from build123d import *

# Parameters (mm, degrees)
F1_DEPTH  = 25.4
F2_W      = 31.608661
F2_H      = 81.88197
F3_DEPTH  = 50.8
F5_DEPTH  = 76.2
F6_W      = 15.80433
F6_H      = 18.276912
F8_W      = 15.80433
F8_H      = 18.276912
F10_R     = 8.263527
F11_DEPTH = 135.636


with BuildPart() as f1:
    # F0 (on Top) → F1 (new body)
    with BuildSketch(Plane.XY):
        with BuildLine():
            Line((45.138903, 75.711831), (26.379006, 75.711831))
            ThreePointArc((26.379006, 75.711831), (-0.25221, 49.080616), (-26.883425, 75.711831))
            Line((-26.883425, 75.711831), (-45.643322, 75.711831))
            Line((-45.643322, 75.711831), (-45.643322, -76.136142))
            Line((-45.643322, -76.136142), (-26.182505, -76.136142))
            ThreePointArc((-26.182505, -76.136142), (-0.25221, -50.205846), (25.678086, -76.136142))
            Line((25.678086, -76.136142), (45.138903, -76.136142))
            Line((45.138903, -76.136142), (45.138903, 75.711831))
        make_face()
        with BuildLine():
            ThreePointArc((-26.883425, 75.711831), (-0.25221, 102.343047), (26.379006, 75.711831))
            Line((26.379006, 75.711831), (45.138903, 75.711831))
            ThreePointArc((45.138903, 75.711831), (-0.25221, 121.102944), (-45.643322, 75.711831))
            Line((-45.643322, 75.711831), (-26.883425, 75.711831))
        make_face()
        with BuildLine():
            ThreePointArc((-45.643322, -76.136142), (-0.25221, -121.527255), (45.138903, -76.136142))
            Line((45.138903, -76.136142), (25.678086, -76.136142))
            ThreePointArc((25.678086, -76.136142), (-0.25221, -102.066438), (-26.182505, -76.136142))
            Line((-26.182505, -76.136142), (-45.643322, -76.136142))
        make_face()
    extrude(amount=F1_DEPTH)

    # F2 (on Top) → F3 (join)
    with BuildSketch(Plane.XY):
        with Locations((0.401416, -2.476901)):
            Rectangle(F2_W, F2_H)
    extrude(amount=F3_DEPTH)

    # F4 (on face) → F5 (cut)
    with BuildSketch(Plane.YZ.offset(16.205747)):
        with BuildLine():
            ThreePointArc((-25.140974, 50.8), (-2.476901, 28.135927), (20.187172, 50.8))
            Line((20.187172, 50.8), (-25.140974, 50.8))
        make_face()
        with BuildLine():
            Line((-25.140974, 50.8), (20.187172, 50.8))
            ThreePointArc((20.187172, 50.8), (-2.476901, 73.464073), (-25.140974, 50.8))
        make_face()
    extrude(amount=-F5_DEPTH, mode=Mode.SUBTRACT)

    # F6 (on face) → F7 (revolve)
    with BuildSketch(Plane.XY.offset(50.8)):
        with Locations((-7.500749, -34.27943)):
            Rectangle(F6_W, F6_H)
    revolve(axis=Axis((0.401416, -34.27943, 50.8), (0, -1, 0)))

    # F8 (on face) → F9 (revolve)
    with BuildSketch(Plane.XY.offset(50.8)):
        with Locations((-7.500749, 29.325628)):
            Rectangle(F8_W, F8_H)
    revolve(axis=Axis((0.401416, 29.325628, 50.8), (0, -1, 0)))

    # F10 (on face) → F11 (cut)
    with BuildSketch(Plane(origin=(0, 38.464084, 0), x_dir=(-1, 0, 0), z_dir=(0, 1, 0))):
        with Locations((-0.401416, 50.8)):
            Circle(F10_R)
    extrude(amount=-F11_DEPTH, mode=Mode.SUBTRACT)


solid = f1.part
The listing builds one solid part. Answer for the finished solid, in the listing's coordinates (mm). A direction names the side the tool comes from. Give positions to 0.01 mm unless a question says otherwise; leave off trailing zeros. Write each loop counter-clockwise with the first axis right and the second up, starting at its lowest first coordinate (ties: lowest second). Pieces come first, ordered by that corner, then holes.
Item 1: Section B-B, the plane x = 23 is taken. Write down the section's boundary in (y, z) (3 decimals), plus the area to 3 significant figures.
Item 2: Section D-D, the plane z = 55.5 is taken. Write down the section's boundary in (x, y).
Item 3: Determine the mould class of faces 1 (the flat face through (-1, 1, 0)), 2 (the cylindrical face through (0.75, 121.09, 12.52)), 3 (the cylindrical face through (5.521, 49.714, 12.522)) for opening direction Y: released by +Y, released by -Y, zero draft, split by the parting line, or undercut.
Item 4: Flat-ended cylindrical pins translate along their axes: P1, Ø12.5, axis at x = -1, z = 55.5, coming from the -Y side; P2, Ø12.5, axis at x = -5.5, z = 57.5, coming from the +Y side; P3, Ø4, axis at x = 7.5, y = -35, coming from the +Z side. Find the tip coordinate at first contact, or state that the pin passes through.
Item 5: Section C-C, the plane y = -86 is taken. Write down the section's boundary in (x, z), plus the area to 3 significant figures.
Item 6: Find the intervals of material crossed by line 1 along Y through (x, z) = (0.5, 60.5); line 2 along X through (y, z) = (27, 50.8); line 3 along Z through (x, y) = (1, 24.5), in increasing order.
Item 7: Which of the six approach directions +Z, -Z, +X, -X, +Y, -Y give full straight-line access (tool end or side, diameter ignored) to faces 4 (the flat face through (-15.403, -3, 27)), 5 (the flat face through (1, 20.187, 60)), 6 (the flat face through (16.206, -3, 27))?
Item 8: Section A-A, the plane z = 33.5 is taken. Write down the section's boundary in (x, y), plus the area to 3 significant figures.
Completed:
1. outline: (-115.119, 0) - (-87.613, 0) - (-87.613, 25.4) - (-115.119, 25.4) - close; (-64.659, 0) - (62.729, 0) - (62.729, 25.4) - (-64.659, 25.4) - close; (88.695, 0) - (114.695, 0) - (114.695, 25.4) - (88.695, 25.4) - close
1. area: 4,590 mm2
2. outline: (-14.69, -43.42) - (-6.4, -43.42) - (-6.4, -25.14) - (-14.69, -25.14) - close; (-14.69, 20.19) - (-6.4, 20.19) - (-6.4, 38.46) - (-14.69, 38.46) - close; (7.2, -43.42) - (15.49, -43.42) - (15.49, -25.14) - (7.2, -25.14) - close; (7.2, 20.19) - (15.49, 20.19) - (15.49, 38.46) - (7.2, 38.46) - close
3. face 1: zero draft
3. face 2: released by +Y
3. face 3: undercut
4. P1: stops at y = -43.42
4. P2: stops at y = 38.46
4. P3: stops at z = 65.76
5. outline: (-44.56, 0) - (-24.23, 0) - (-24.23, 25.4) - (-44.56, 25.4) - close; (23.73, 0) - (44.05, 0) - (44.05, 25.4) - (23.73, 25.4) - close
5. area: 1,030 mm2
6. line 1: y = -43.42 to -25.14, 20.19 to 38.46
6. line 2: x = -15.4 to -7.86, 8.66 to 16.21
6. line 3: z = 0 to 42.56, 59.04 to 66.59
7. face 4: +Z, -X, +Y, -Y
7. face 5: +Z, +X, -X
7. face 6: +Z, +X, +Y, -Y
8. outline: (-15.4, -43.42) - (16.21, -43.42) - (16.21, -17.12) - (-15.4, -17.12) - close; (-15.4, 12.16) - (16.21, 12.16) - (16.21, 38.46) - (-15.4, 38.46) - close
8. area: 1,660 mm2
